Autodesk Inventor part; units mm, degrees
ref_plane "YZ Plane" through (0, 0, 0) normal (1, 0, 0) x (0, 1, 0)
ref_plane "XZ Plane" through (0, 0, 0) normal (0, 1, 0) x (-1, 0, 0)
ref_plane "XY Plane" through (0, 0, 0) normal (0, 0, 1) x (1, 0, 0)
sketch "スケッチ1" plane through (0, 0, 0) normal (0, 0, 1) x (1, 0, 0)
  line L0 (-23.7126, 8.7959) -> (24.2874, 8.7959)
  line L1 (24.2874, 8.7959) -> (24.2874, -1.2041)
  line L2 (24.2874, -1.2041) -> (-23.7126, -1.2041)
  line L3 (-23.7126, -1.2041) -> (-23.7126, 8.7959)
  point P0 (0, 0)
  dimension "d0" = 48
  dimension "d1" = 10
extrude "押し出し1" add sketch "スケッチ1" along normal blind 3
sketch "スケッチ2" plane through (0, 0, 3) normal (0, 0, 1) x (1, 0, 0)
  line L0 (-15.7126, 3.7959) -> (-0.7126, 3.7959) construction
  line L1 (-15.7126, 2.2959) -> (-0.7126, 2.2959)
  line L2 (-0.7126, 5.2959) -> (-15.7126, 5.2959)
  arc A0 (-15.7126, 5.2959) -> (-15.7126, 2.2959) centre (-15.7126, 3.7959) ccw
  arc A1 (-0.7126, 2.2959) -> (-0.7126, 5.2959) centre (-0.7126, 3.7959) ccw
  line L3 (-23.7126, 8.7959) -> (-23.7126, -1.2041)
  line L4 (24.2874, 8.7959) -> (-23.7126, 8.7959)
  point P0 (0, 0)
  point P1 (-8.2126, 3.7959)
  dimension "d4" = 15
  dimension "d5" = 3
  dimension "d6" = 8
  dimension "d7" = 5
extrude "押し出し2" cut sketch "スケッチ2" against normal blind 3
properties part number "creat7"
Input: part model. Units: mm. Frame: model coordinates. A direction names the side the tool comes from. Round coordinates to 2 decimals unless told otherwise and drop trailing zeros. Loops run counter-clockwise (first coordinate to the right, second up) from the corner with the lowest first, then second, coordinate; pieces in that order, holes last.
1) Section query B-B on y = 3.75. Return the cut outline in (x, z).
Ans:
outline: (-23.71, 0) - (-17.21, 0) - (-17.21, 3) - (-23.71, 3) - close; (0.79, 0) - (24.29, 0) - (24.29, 3) - (0.79, 3) - close
2) Pull-direction query (X, two-part tool) for faces 1 (the flat face through (-8, 2.296, 2)), 2 (the cylindrical face through (-17.212, 3.829, 1.521)), 3 (the flat face through (0, 6, 3)), 4 (the flat face through (24.287, 4, 1)); classes: released by +X, released by -X, zero draft, split by the parting line, or undercut.
Ans:
face 1: undercut
face 2: undercut
face 3: zero draft
face 4: released by +X
3) Set-up query: faces 5 (the cylindrical face through (0.787, 3.763, 1.521)), 6 (the flat face through (0, 8.796, 1)). Return all of +Z, -Z, +X, -X, +Y, -Y with unobstructed straight access to the full face (end or side cutting, diameter ignored); none if empty.
Ans:
face 5: +Z, -Z
face 6: +Z, -Z, +X, -X, +Y
4) Section query C-C on z = 1.3. Return the cut outline in (x, y).
Ans:
outline: (-23.71, -1.2) - (24.29, -1.2) - (24.29, 8.8) - (-23.71, 8.8) - close; hole (-15.71, 2.3) - (-0.71, 2.3) arc R1.5 ccw to (-0.71, 5.3) - (-15.71, 5.3) arc R1.5 ccw to start
5) Section query A-A on x = -3.5. Return the cut outline in (y, z), plus the area to 3 significant figures.
Ans:
outline: (-1.2, 0) - (2.3, 0) - (2.3, 3) - (-1.2, 3) - close; (5.3, 0) - (8.8, 0) - (8.8, 3) - (5.3, 3) - close
area: 21.0 mm2
6) Material intervals for line 1 (Y direction, x = -9.5, z = 0.3); line 2 (X direction, y = 5, z = 2.8); line 3 (X direction, y = 3.5, z = 2.55), sorted ascending.
Ans:
line 1: y = -1.2 to 2.3, 5.3 to 8.8
line 2: x = -23.71 to -16.61, 0.18 to 24.29
line 3: x = -23.71 to -17.18, 0.76 to 24.29
